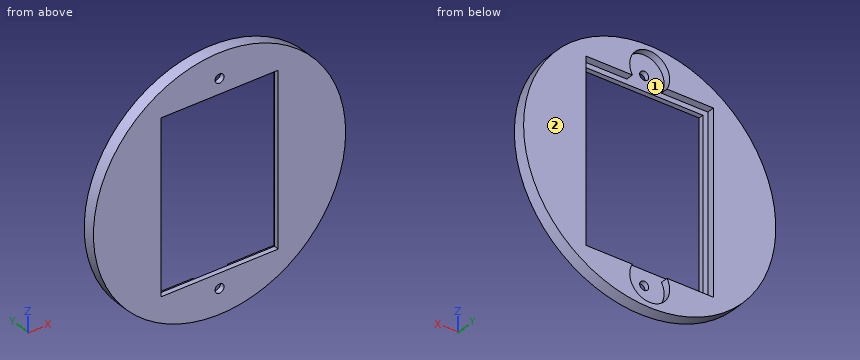
```python
from build123d import *

# Parameters (mm, degrees)
SKETCH1_R           = 25.25
BOSS_EXTRUDE1_DEPTH = 2.5
SKETCH2_W           = 25.5
SKETCH2_H           = 36.5
CUT_EXTRUDE1_DEPTH  = 1.5
SKETCH3_W           = 23.5
SKETCH3_H           = 34.5
CUT_EXTRUDE2_DEPTH  = 1.2
SKETCH4_R           = 4
CUT_EXTRUDE3_DEPTH  = 1.5
SKETCH5_R           = 0.9
CUT_EXTRUDE4_DEPTH  = 2


with BuildPart() as part:
    # Sketch1 → Boss-Extrude1 (new body)
    with BuildSketch(Plane(origin=(0, 0, 0), x_dir=(1, 0, 0), z_dir=(0, 1, 0))):
        Circle(SKETCH1_R)
    extrude(amount=BOSS_EXTRUDE1_DEPTH)

    # Sketch2 → Cut-Extrude1 (cut)
    with BuildSketch(Plane(origin=(0, 2.5, 0), x_dir=(1, 0, 0), z_dir=(0, 1, 0))):
        Rectangle(SKETCH2_W, SKETCH2_H)
    extrude(amount=-CUT_EXTRUDE1_DEPTH, mode=Mode.SUBTRACT)

    # Sketch3 → Cut-Extrude2 (cut)
    with BuildSketch(Plane(origin=(0, 1, 0), x_dir=(1, 0, 0), z_dir=(0, 1, 0))):
        Rectangle(SKETCH3_W, SKETCH3_H)
    extrude(amount=-CUT_EXTRUDE2_DEPTH, mode=Mode.SUBTRACT)

    # Sketch4 → Cut-Extrude3 (cut)
    with BuildSketch(Plane(origin=(0, 2.5, 0), x_dir=(1, 0, 0), z_dir=(0, 1, 0))):
        with Locations((0, 20.25)):
            Circle(SKETCH4_R)
        with Locations((0, -20.25)):
            Circle(SKETCH4_R)
    extrude(amount=-CUT_EXTRUDE3_DEPTH, mode=Mode.SUBTRACT)

    # Sketch5 → Cut-Extrude4 (cut, through all)
    with BuildSketch(Plane(origin=(0, 1, 0), x_dir=(1, 0, 0), z_dir=(0, 1, 0))):
        with Locations((0, 20.25)):
            Circle(SKETCH5_R)
        with Locations((0, -20.25)):
            Circle(SKETCH5_R)
    extrude(amount=-CUT_EXTRUDE4_DEPTH, mode=Mode.SUBTRACT)


solid = part.part
```
CAD build for the part. Positions are in the model's coordinates, mm. Face numbers are marked on the shaded views. Coordinates: 2 decimals unless noted, no trailing zeros. Order: outer loops, then holes, each group sorted by start corner. A loop starts at its lowest first (then second) coordinate and runs counter-clockwise, first axis right, second up. Notation, with made-up numbers: (13.5, 81.25) - (65.5, 81.25) arc R25 ccw to (65.5, 117.25) - close; hole circle Ø4 at (39, 1). An arc over 180 degrees is marked (long way). Answer in a Markdown table with one row per item.
1. Slice it at A-A, the plane x = 0. List the corners of the cut face in (y, z), then the cut area to 3 significant figures.
Answer:
| item | result |
|---|---|
| outline | (0, -25.25) - (2.5, -25.25) - (2.5, -24.25) - (1, -24.25) - (1, -21.15) - (0, -21.15) - close; (0, -19.35) - (1, -19.35) - (1, -17.25) - (0, -17.25) - close; (0, 17.25) - (1, 17.25) - (1, 19.35) - (0, 19.35) - close; (0, 21.15) - (1, 21.15) - (1, 24.25) - (2.5, 24.25) - (2.5, 25.25) - (0, 25.25) - close |
| area | 15.4 mm² |
2. Slice it at D-D, the plane x = 7. List the corners of the cut face in (y, z), then the cut area to 3 significant figures.
Answer:
| item | result |
|---|---|
| outline | (0, -24.26) - (2.5, -24.26) - (2.5, -18.25) - (1, -18.25) - (1, -17.25) - (0, -17.25) - close; (0, 17.25) - (1, 17.25) - (1, 18.25) - (2.5, 18.25) - (2.5, 24.26) - (0, 24.26) - close |
| area | 32.1 mm² |
3. Flat gauge pins, fed straight in: P1, Ø0.8, axis at x = 2, y = 0.5, coming from the +Z side; P2, Ø3, axis at x = 0, z = 20.25, coming from the +Y side; P3, Ø0.8, axis at x = 7, y = 2, coming from the +Z side. Where does each tip first touch, or does it go through?
Answer:
| item | result |
|---|---|
| P1 | z = 25.2 |
| P2 | y = 1 |
| P3 | z = 24.37 |
4. Slice it at B-B, the plane y = 0.4. List the corners of the cut face in (x, z), then the cut area to 3 significant figures.
Answer:
| item | result |
|---|---|
| outline | circle Ø50.5 at (0, 0); hole (-11.75, -17.25) - (11.75, -17.25) - (11.75, 17.25) - (-11.75, 17.25) - close; hole circle Ø1.8 at (0, -20.25); hole circle Ø1.8 at (0, 20.25) |
| area | 1,190 mm² |
5. Drill centre lines: L1, parallel to Z at x = 0, y = 0.4; L2, parallel to X at y = 2.2, z = -7.5; L3, parallel to X at y = 2.15, z = -7. Where is each one in solid material? Low to high. Write a range as from..to.
Answer:
| item | result |
|---|---|
| L1 | -25.25..-21.15, -19.35..-17.25, 17.25..19.35, 21.15..25.25 |
| L2 | -24.11..-12.75, 12.75..24.11 |
| L3 | -24.26..-12.75, 12.75..24.26 |
6. Slice it at C-C, the plane z = 0. List the corners of the cut face in (x, y).
Answer:
| item | result |
|---|---|
| outline | (-25.25, 0) - (-11.75, 0) - (-11.75, 1) - (-12.75, 1) - (-12.75, 2.5) - (-25.25, 2.5) - close; (11.75, 0) - (25.25, 0) - (25.25, 2.5) - (12.75, 2.5) - (12.75, 1) - (11.75, 1) - close |
7. Pull direction X, two halves, no side cores. Call the marked faces 1 and 2: +X half, -X half, draft (parallel to the pull), parting line (faces both ways), or undercut.
Answer:
| item | result |
|---|---|
| face 1 | undercut |
| face 2 | draft |
